Could you check a few things on this drawing? It's one solid part, dimensions in mm from its lowest x, y, z. A direction names the side the tool comes from. Coordinates: 2 decimals unless noted, no trailing zeros. Answer as a JSON object with one key per item and string values. Group by question number.
Item 1: Which directions (+Z, -Z, +X, -X, +Y, -Y) give clear straight access to the entire face, cutting with the end or side of a thin tool? Please do the marked faces 1, 2 and 3.
Item 2: Suppose I cut it at B-B (y = 12). Count the separate pieces of the cut face and the enclosed holes in it, then the cut area to 3 significant figures.
Item 3: We'd pull the mould along X, two halves only. Please class the marked faces 4, 5 and 6: +X half, -X half, draft (parallel to the pull), parting line (faces both ways), or undercut.
Item 4: If I drill on line 1 (Z direction, x = 25.4, y = 23.5) (1 decimal); line 2 (Z direction, x = 30, y = 22.5); line 3 (Z direction, x = 5, y = 16), over which ranges is the centre line in solid material (lowest first)?
Item 5: I'm going to push flat-ended pins straight in: pin 1 Ø1 at (y, z) = (18, 10) entering from -X; pin 2 Ø4 at (x, y) = (33.5, 5.5) entering from -Z; pin 3 Ø1.5 at (x, y) = (14, 5.5) entering from -Z. Where does each tip first touch, or does it pass through?
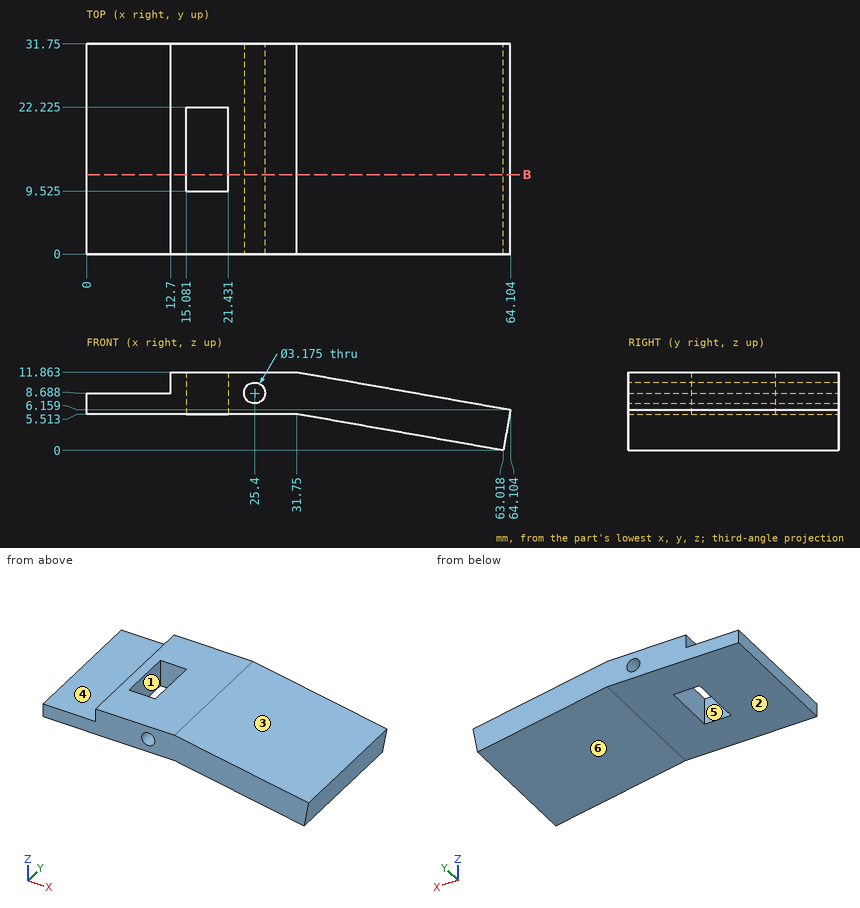
From the geometry:
{
 "1": {"face 1": "+Z, -Z", "face 2": "-Z, -X, +Y, -Y", "face 3": "+Z, +X, +Y, -Y"},
 "2": {"separate pieces": "2", "enclosed holes": "1", "area": "315 mm2"},
 "3": {"face 4": "draft", "face 5": "undercut", "face 6": "-X half"},
 "4": {"line 1": "5.5 to 7.1, 10.3 to 11.9", "line 2": "5.51 to 11.86", "line 3": "5.51 to 8.69"},
 "5": {"pin 1": "x = 12.7", "pin 2": "z = 4.85", "pin 3": "z = 5.51"}
}
